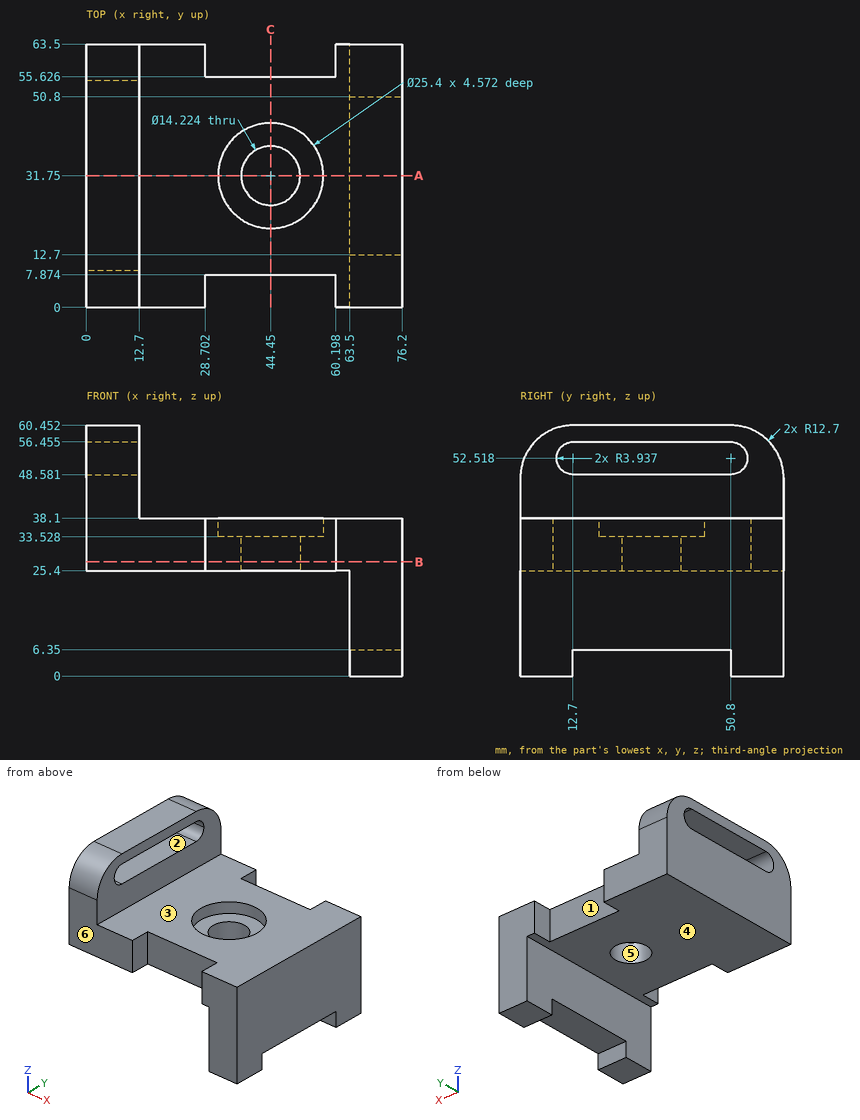
Can you work these out from the drawing? Everything is in mm from the part's minimum corner. A direction names the side the tool comes from. Coordinates: 2 decimals unless noted, no trailing zeros. Loops run counter-clockwise (first coordinate to the right, second up) from the corner with the lowest first, then second, coordinate; pieces in that order, holes last. Notation, with made-up numbers: M -33.5,27 L -6.5,27 A26 cw -6.5,50 Z; hole C 41,25 d3. An arc over 180 degrees is marked long. One line per item, written item: value.
1. Imagine slicing it at C-C (x = 44.45). List the corners of the cut face in (y, z) for me, and give its area (3 significant figures).
Geometry says:
outline: M 7.87,25.4 L 24.64,25.4 L 24.64,33.53 L 19.05,33.53 L 19.05,38.1 L 7.87,38.1 Z; M 38.86,25.4 L 55.63,25.4 L 55.63,38.1 L 44.45,38.1 L 44.45,33.53 L 38.86,33.53 Z
area: 375 mm2
2. Imagine slicing it at A-A (y = 31.75). State how many separate pieces and enclosed holes the cut face has, and give its area (3 significant figures).
Geometry says:
separate pieces: 3
enclosed holes: 0
area: 1,160 mm2
3. Please list where these lines run through material, in increasing order: probe 1 along Z at (x, y) = (10.5, 23) (1 decimal); probe 2 along Y at (x, z) = (44.45, 37.15); probe 3 along Y at (x, z) = (44, 28).
Geometry says:
probe 1: z = 25.4 to 48.6, 56.5 to 60.5
probe 2: y = 7.87 to 19.05, 44.45 to 55.63
probe 3: y = 7.87 to 24.65, 38.85 to 55.63
4. On a 3-axis mill with a long thin cutter (end or side, diameter ignored), from which of +Z, -Z, +X, -X, +Y, -Y can I reach the whole of each face in a straight line? I mean the marked faces 1, 2 and 3. Say none if no direction works.
Geometry says:
face 1: +Z, -Z, +Y
face 2: +X, -X
face 3: +Z, +X, +Y, -Y
5. Will these pins go through, and if not, where does the flat tip stop? pin 1 Ø10 at (x, z) = (47.5, 33.5) entering from +Y; pin 2 Ø5 at (x, z) = (39, 37) entering from -Y; pin 3 Ø2.5 at (y, z) = (58.5, 31) entering from -X; pin 4 Ø23 at (x, y) = (44.45, 31.75) entering from +Z.
Geometry says:
pin 1: stops at y = 55.63
pin 2: stops at y = 7.87
pin 3: stops at x = 0
pin 4: stops at z = 33.53
6. Thinking about a two-plate mould opening in Y: for the marked faces 4, 5 and 6, which applies, +Y half, -Y half, draft (parallel to the pull), parting line (faces both ways), or undercut?
Geometry says:
face 4: draft
face 5: undercut
face 6: -Y half
7. Imagine slicing it at B-B (z = 27.5). List the corners of the cut face in (x, y) for me, and give its area (3 significant figures).
Geometry says:
outline: M 0,0 L 28.7,0 L 28.7,7.87 L 60.2,7.87 L 60.2,0 L 76.2,0 L 76.2,63.5 L 60.2,63.5 L 60.2,55.63 L 28.7,55.63 L 28.7,63.5 L 0,63.5 Z; hole C 44.45,31.75 d14.22
area: 4,180 mm2
